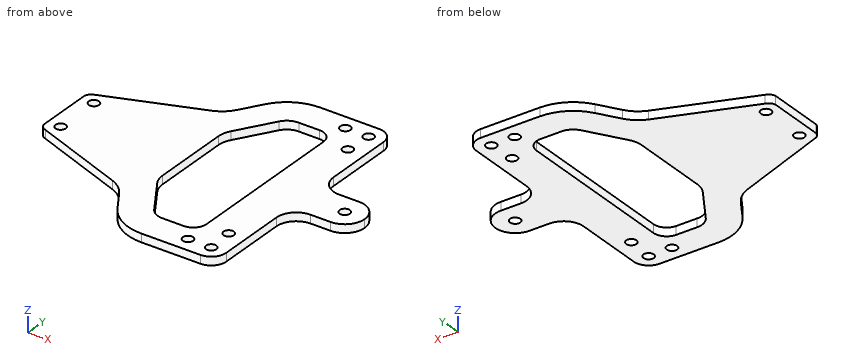
from build123d import *

# Parameters (mm, degrees)
F0_R     = 1.55
F1_DEPTH = 2.5


# Not quite as in the source:
# - ends of sketch curves that miss each other by under 0.0002 mm in the source are joined


with BuildPart() as f1:
    # F0 (on Top) → F1 (new body)
    with BuildSketch(Plane.XY):
        with BuildLine():
            Line((24.1317584196, 12.0030992724), (24.1317584196, 33.007258608))
            ThreePointArc((24.1317584196, 33.007258608), (22.8094861978, 36.1776713218), (19.6355297089, 37.4914143753))
            Line((19.6355297089, 37.4914143753), (1.8379933168, 37.5062195629))
            ThreePointArc((1.8379933168, 37.5062195629), (-4.952633867, 35.7733094677), (-10.0545165801, 30.9684798423))
            Line((-10.0545165801, 30.9684798423), (-13.9594315472, 24.7955182975))
            ThreePointArc((-13.9594315472, 24.7955182975), (-16.1001567778, 22.383955311), (-18.8970513925, 20.7790499976))
            Line((-18.8970513925, 20.7790499976), (-46.5253097099, 10.4110515716))
            ThreePointArc((-46.5253097099, 10.4110515716), (-47.6965598622, 9.7014043841), (-48.3182136925, 8.4811697487))
            Line((-48.3182136925, 8.4811697487), (-48.3182136925, -8.4811697487))
            ThreePointArc((-48.3182136925, -8.4811697487), (-47.6965598622, -9.7014043841), (-46.5253097099, -10.4110515716))
            Line((-46.5253097099, -10.4110515716), (-18.8970513925, -20.7790499976))
            ThreePointArc((-18.8970513925, -20.7790499976), (-16.1001567778, -22.383955311), (-13.9594315472, -24.7955182975))
            Line((-13.9594315472, -24.7955182975), (-10.0545165801, -30.9684798423))
            ThreePointArc((-10.0545165801, -30.9684798423), (-4.952633867, -35.7733094677), (1.8379933168, -37.5062195629))
            Line((1.8379933168, -37.5062195629), (19.635501821, -37.4914143985))
            ThreePointArc((19.635501821, -37.4914143985), (22.8150621521, -36.1720727032), (24.1317584196, -32.9914159555))
            Line((24.1317584196, -32.9914159555), (24.1317584196, -12.0030992724))
            Line((24.1317584196, -12.0030992724), (24.1317584196, -12))
            ThreePointArc((24.1317584196, -12), (25.8891177325, -7.7573593129), (30.1317584196, -6))
            Line((30.1317584196, -6), (36.1317584196, -6))
            ThreePointArc((36.1317584196, -6), (40.3733032071, -4.2437363038), (42.1317576192, -0.003099272))
            Line((42.1317576192, -0.003099272), (42.1317584196, 0))
            ThreePointArc((42.1317584196, 0), (40.3743991067, 4.2426406871), (36.1317584196, 6))
            Line((36.1317584196, 6), (30.1317584196, 6))
            ThreePointArc((30.1317584196, 6), (25.8891177325, 7.7573593129), (24.1317584196, 12))
            Line((24.1317584196, 12), (24.1317584196, 12.0030992724))
        make_face()
        with Locations((-44.3682136925, -7)):
            Circle(F0_R, mode=Mode.SUBTRACT)
        with Locations((12.6317863075, -32.997239003)):
            Circle(F0_R, mode=Mode.SUBTRACT)
        with Locations((19.1317584196, -25)):
            Circle(F0_R, mode=Mode.SUBTRACT)
        with Locations((19.6317863075, -32.9914159323)):
            Circle(F0_R, mode=Mode.SUBTRACT)
        with Locations((-44.3682136925, 7)):
            Circle(F0_R, mode=Mode.SUBTRACT)
        with BuildLine():
            Line((-9.2339508783, 15.4306240067), (-2.4342503505, 26.1797159146))
            ThreePointArc((-2.4342503505, 26.1797159146), (-0.5889861734, 27.9038009834), (1.8634800061, 28.5061952445))
            Line((1.8634800061, 28.5061952445), (8.1350890009, 28.5009780993))
            ThreePointArc((8.1350890009, 28.5009780993), (10.9631282223, 27.3264639859), (12.1317584196, 24.4959882833))
            Line((12.1317584196, 24.4959882833), (12.1317584196, -24.5019407212))
            ThreePointArc((12.1317584196, -24.5019407212), (10.9611450551, -27.3294080096), (8.1344727862, -28.5019398002))
            Line((8.1344727862, -28.5019398002), (1.8634800061, -28.5061952445))
            ThreePointArc((1.8634800061, -28.5061952445), (-0.5889861734, -27.9038009834), (-2.4342503505, -26.1797159146))
            Line((-2.4342503505, -26.1797159146), (-9.2339508783, -15.4306240067))
            ThreePointArc((-9.2339508783, -15.4306240067), (-10.0416860208, -13.6364803831), (-10.3182136925, -11.688424981))
            Line((-10.3182136925, -11.688424981), (-10.3182136925, 11.688424981))
            ThreePointArc((-10.3182136925, 11.688424981), (-10.0416860208, 13.6364803831), (-9.2339508783, 15.4306240067))
        make_face(mode=Mode.SUBTRACT)
        with Locations((36.1317584196, 0)):
            Circle(F0_R, mode=Mode.SUBTRACT)
        with Locations((19.1317584196, 25)):
            Circle(F0_R, mode=Mode.SUBTRACT)
        with Locations((12.6317863075, 32.997239003)):
            Circle(F0_R, mode=Mode.SUBTRACT)
        with Locations((19.6317863075, 32.9914159323)):
            Circle(F0_R, mode=Mode.SUBTRACT)
    extrude(amount=F1_DEPTH)


solid = f1.part
Can you work these out from the model? Positions are in its coordinate system, mm. Coordinates: 2 decimals unless noted, no trailing zeros. Write each loop counter-clockwise with the first axis right and the second up, starting at its lowest first coordinate (ties: lowest second). Pieces come first, ordered by that corner, then holes. Notation, with made-up numbers: (44, 3) -> (101, 3) arc R21 ccw to (101, 25) -> close; hole circle Ø4 at (-23.75, 22). An arc over 180 degrees is marked (long way). Answer as CSV lines item,"result".
1) If we section it at D-D on x = -39.5: Please give me the cut outline in (y, z), then the cut area to 3 significant figures.
Check result:
outline,"(-13.05, 0) -> (13.05, 0) -> (13.05, 2.5) -> (-13.05, 2.5) -> close"
area,"65.2 mm²"
2) If we section it at C-C on z = 1.35: Count the separate pieces of the cut face and the enclosed holes in it, then the cut area to 3 significant figures.
Check result:
separate pieces,"1"
enclosed holes,"10"
area,"2,860 mm²"
3) Will these pins go through, and if not, where does the flat tip stop? P1, Ø1, axis at y = -9, z = 2, coming from the -X side; P2, Ø1.5, axis at y = 26.5, z = 1.5, coming from the +X side; P3, Ø0.8, axis at x = 32.5, z = 2, coming from the +Y side.
Check result:
P1,"x = -48.31"
P2,"x = 24.13"
P3,"y = 6"
4) If we section it at B-B on y = 3: Please give me the cut outline in (x, z), then the cut area to 3 significant figures.
Check result:
outline,"(-48.32, 0) -> (-10.32, 0) -> (-10.32, 2.5) -> (-48.32, 2.5) -> close; (12.13, 0) -> (41.33, 0) -> (41.33, 2.5) -> (12.13, 2.5) -> close"
area,"168 mm²"
5) If we section it at A-A on x = -6.5: Please give me the cut outline in (y, z), then the cut area to 3 significant figures.
Check result:
outline,"(-34.79, 0) -> (-19.75, 0) -> (-19.75, 2.5) -> (-34.79, 2.5) -> close; (19.75, 0) -> (34.79, 0) -> (34.79, 2.5) -> (19.75, 2.5) -> close"
area,"75.2 mm²"
6) If I drill on line 1 (Y direction, x = 4.5, z = 0.15); line 2 (Y direction, x = 13.5, z = 0.6); line 3 (X direction, y = 0.5, z = 1.65), over which ranges is the centre line in solid material (lowest first)? Write a range as from..to.
Check result:
line 1,"-37.5..-28.5, 28.5..37.5"
line 2,"-37.5..-34.28, -31.71..31.71, 34.28..37.5"
line 3,"-48.32..-10.32, 12.13..34.66, 37.6..42.11"
